Check sheet for the drawn part. Datum: minimum x, y, z corner. Units: mm. A direction names the side the tool comes from. Give positions to 0.01 mm unless a question says otherwise; leave off trailing zeros. Order: outer loops, then holes, each group sorted by start corner. A loop starts at its lowest first (then second) coordinate and runs counter-clockwise, first axis right, second up. Notation, with made-up numbers: M -25.75,-26 L -7.75,-26 A24 ccw -7.75,8 Z; hole C 22,21 d9. An arc over 180 degrees is marked long. Put each result on its own line as item: value. Start each with the question number.
Q1. Material ranges on L1, parallel to X at y = 85, z = 8.8; L2, parallel to Y at x = 5, z = 8.1; L3, parallel to Y at x = 120, z = 8.15, recorded low to high.
Q2. Section check C-C on z = 4. Record the cut outline in (x, y), then the cut area to 4 significant figures.
Q3. Section check A-A on x = 120. Record the cut outline in (y, z).
Q4. Go/stop test with flat-tipped pins: pin 1 (3 mm diameter, centred on y = 44.5, z = 4.5, fed in from -X); pin 2 (3 mm diameter, centred on x = 5, y = 85, fed in from +Z); pin 3 (3 mm diameter, centred on x = 6, y = 7, fed in from -Z); pin 4 (4 mm diameter, centred on x = 89, z = 1.5, fed in from -Y). Record where each tip stops, or that it passes through.
Q5. Section check B-B on x = 5. Record the cut outline in (y, z), then the cut area to 3 significant figures.
Q6. Access from +Z, -Z, +X, -X, +Y, -Y to the whole of each face (thin tool, end or side, straight path). Record for the marked faces 1 and 2.
Q7. Mould release check, pull along X, two halves, no side actions. Record for the marked faces 3 and 4: +X half, -X half, draft (parallel to the pull), parting line (faces both ways), or undercut.
Q8. Section check D-D on y = 33. Record the cut outline in (x, z), then the cut area to 3 significant figures.
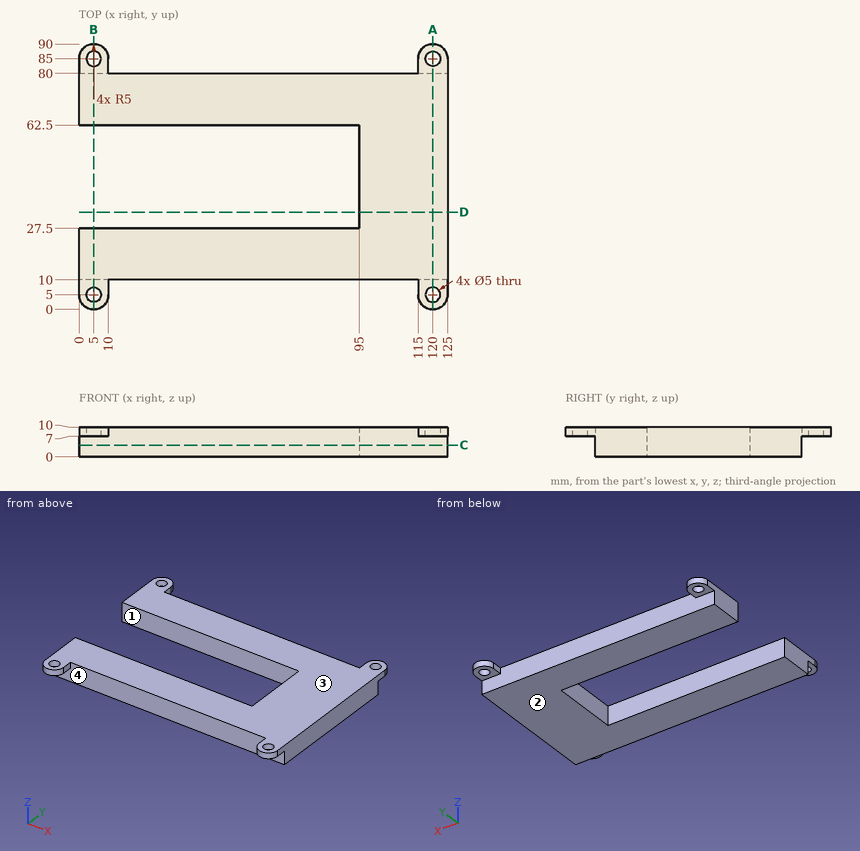
Results found:
1. L1: x = 0 to 2.5, 7.5 to 10, 115 to 117.5, 122.5 to 125
1. L2: y = 0 to 2.5, 7.5 to 27.5, 62.5 to 82.5, 87.5 to 90
1. L3: y = 0 to 2.5, 7.5 to 82.5, 87.5 to 90
2. outline: M 0,10 L 125,10 L 125,80 L 0,80 L 0,62.5 L 95,62.5 L 95,27.5 L 0,27.5 Z
2. area: 5,425 mm^2
3. outline: M 0,7 L 2.5,7 L 2.5,10 L 0,10 Z; M 7.5,7 L 10,7 L 10,0 L 80,0 L 80,7 L 82.5,7 L 82.5,10 L 7.5,10 Z; M 87.5,7 L 90,7 L 90,10 L 87.5,10 Z
4. pin 1: stops at x = 95
4. pin 2: passes through
4. pin 3: stops at z = 7
4. pin 4: stops at y = 10
5. outline: M 0,7 L 2.5,7 L 2.5,10 L 0,10 Z; M 7.5,7 L 10,7 L 10,0 L 27.5,0 L 27.5,10 L 7.5,10 Z; M 62.5,0 L 80,0 L 80,7 L 82.5,7 L 82.5,10 L 62.5,10 Z; M 87.5,7 L 90,7 L 90,10 L 87.5,10 Z
5. area: 380 mm^2
6. face 1: +Z, -Z, -X
6. face 2: -Z, +X, -X, +Y, -Y
7. face 3: draft
7. face 4: undercut
8. outline: M 95,0 L 125,0 L 125,10 L 95,10 Z
8. area: 300 mm^2
